```python
from build123d import *

# Parameters (mm, degrees)
SALIENTE_EXTRUIR1_DEPTH = 88.9
CROQUIS2_W              = 38.1
CROQUIS2_H              = 4.7625
CROQUIS2_W_2            = 4.7625
CROQUIS2_H_2            = 38.1
SALIENTE_EXTRUIR2_DEPTH = 76.2
CROQUIS4_R              = 6.35
CORTAR_EXTRUIR2_DEPTH   = 77.8
CROQUIS5_R              = 6.35
CORTAR_EXTRUIR3_DEPTH   = 77.8


with BuildPart() as part:
    # Croquis1 → Saliente-Extruir1 (new, symmetric)
    with BuildSketch(Plane.XY):
        Polygon((0, 31.75), (0, -31.75), (76.2, -31.75), (76.2, -26.9875), (4.7625, -26.9875), (4.7625, 26.9875), (76.2, 26.9875), (76.2, 31.75), align=None)
    extrude(amount=SALIENTE_EXTRUIR1_DEPTH, both=True)

    # Croquis2 → Saliente-Extruir2 (add, through all)
    with BuildSketch(Plane(origin=(0, 0, 0), x_dir=(0, 0, -1), z_dir=(1, 0, 0))):
        with Locations((-65.0875, 34.13125)):
            Rectangle(CROQUIS2_W, CROQUIS2_H)
        with Locations((-86.51875, 50.8)):
            Rectangle(CROQUIS2_W_2, CROQUIS2_H_2)
    saliente_extruir2 = extrude(amount=SALIENTE_EXTRUIR2_DEPTH)

    # Croquis4 → Cortar-Extruir2 (cut)
    with BuildSketch(Plane(origin=(0, 0, 84.1375), x_dir=(-1, 0, 0), z_dir=(0, 0, -1))):
        with Locations(Location((-38.1, 53.18125, 0), (0, 0, 90))):
            Circle(CROQUIS4_R)
    cortar_extruir2 = extrude(amount=-CORTAR_EXTRUIR2_DEPTH, mode=Mode.SUBTRACT)

    # Simetría3: Saliente-Extruir2, Cortar-Extruir2 across plane
    add(saliente_extruir2.mirror(Plane.ZX))
    add(cortar_extruir2.mirror(Plane.ZX), mode=Mode.SUBTRACT)

    # Croquis5 → Cortar-Extruir3 (cut)
    with BuildSketch(Plane(origin=(0, -31.75, 0), x_dir=(-1, 0, 0), z_dir=(0, -1, 0))):
        with Locations(Location((-56.2, 68.9, 0), (0, 0, 180))):
            Circle(CROQUIS5_R)
    extrude(amount=-CORTAR_EXTRUIR3_DEPTH, mode=Mode.SUBTRACT)


solid = part.part
```
For this review, take the finished solid that the model builds, in its own axes (mm). A direction names the side the tool comes from. Round coordinates to 2 decimals unless told otherwise and drop trailing zeros. Write each loop counter-clockwise with the first axis right and the second up, starting at its lowest first coordinate (ties: lowest second). Pieces come first, ordered by that corner, then holes. Notation, with made-up numbers: (62.5, -4.5) - (104.5, -4.5) arc R8 ccw to (104.5, -0.5) - close; hole circle Ø7 at (-1, 50). An arc over 180 degrees is marked (long way). Put each result on its own line as item: value.
Q1. We need section C-C (x = 21). Give the boundary of the cut face in (y, z).
Solved:
outline: (-69.85, 84.14) - (-36.51, 84.14) - (-36.51, 46.04) - (-31.75, 46.04) - (-31.75, -88.9) - (-26.99, -88.9) - (-26.99, 88.9) - (-69.85, 88.9) - close; (26.99, -88.9) - (31.75, -88.9) - (31.75, 46.04) - (36.51, 46.04) - (36.51, 84.14) - (69.85, 84.14) - (69.85, 88.9) - (26.99, 88.9) - close
Q2. Insertion check: pin 1 Ø5 at (x, y) = (22, 47.5) entering from -Z; pin 2 Ø6 at (x, z) = (36, -54) entering from +Y; pin 3 Ø23 at (x, z) = (35.5, -20.5) entering from -Y; pin 4 Ø12 at (y, z) = (8, -43) entering from -X. Each pin has a flat end and moves straight along its axis. Give the tip position at first contact, or say it passes through.
Solved:
pin 1: stops at z = 84.14
pin 2: stops at y = 31.75
pin 3: stops at y = -31.75
pin 4: stops at x = 0
Q3. Machinability: for faces 4 (the face through (39, 31.75, -20)), 5 (the face through (76.2, 31, 27)), 6 (the face through (38, -60, 84.138)), 7 (the face through (41, -26.988, 1)), which of the approach directions +Z, -Z, +X, -X, +Y, -Y give a long, thin tool a straight path to every point of the face, cutting with its end or side? Answer none if there is none.
Solved:
face 4: -Z, +X, -X, +Y
face 5: +Z, -Z, +X, +Y, -Y
face 6: -Z, +X, -X, -Y
face 7: +Z, -Z, +X
Q4. We need section A-A (x = 56.2). Give the boundary of the cut face in (y, z), and give its area (3 significant figures).
Solved:
outline: (-69.85, 84.14) - (-36.51, 84.14) - (-36.51, 46.04) - (-31.75, 46.04) - (-31.75, -62.55) - (-26.99, -62.55) - (-26.99, 88.9) - (-69.85, 88.9) - close; (-31.75, -88.9) - (-26.99, -88.9) - (-26.99, -75.25) - (-31.75, -75.25) - close; (26.99, -88.9) - (31.75, -88.9) - (31.75, -75.25) - (26.99, -75.25) - close; (26.99, -62.55) - (31.75, -62.55) - (31.75, 46.04) - (36.51, 46.04) - (36.51, 84.14) - (69.85, 84.14) - (69.85, 88.9) - (26.99, 88.9) - close
area: 2,300 mm2
Q5. Wall thickness on probe 1 along Y at (x, z) = (39, -19.5); probe 2 along Z at (x, y) = (56.2, 29.95); probe 3 along Y at (x, z) = (70, 55): over which ranges is each line inside the solid? List them lowest first.
Solved:
probe 1: y = -31.75 to -26.99, 26.99 to 31.75
probe 2: z = -88.9 to -75.25, -62.55 to 88.9
probe 3: y = -36.51 to -26.99, 26.99 to 36.51
Q6. We need section D-D (z = -48). Give the boundary of the cut face in (x, y).
Solved:
outline: (0, -31.75) - (76.2, -31.75) - (76.2, -26.99) - (4.76, -26.99) - (4.76, 26.99) - (76.2, 26.99) - (76.2, 31.75) - (0, 31.75) - close
Q7. Mouldability with a two-part tool opening along Y and no side actions: class faces 1 (the face through (0, -1, 1)), 2 (the face through (40, 26.988, 1)), 3 (the face through (38, 36.512, 65)) as released by +Y, released by -Y, zero draft, split by the parting line, or undercut.
Solved:
face 1: zero draft
face 2: undercut
face 3: released by +Y
Q8. We need section B-B (z = -68.9). Give the boundary of the cut face in (x, y).
Solved:
outline: (0, -31.75) - (49.85, -31.75) - (49.85, -26.99) - (4.76, -26.99) - (4.76, 26.99) - (49.85, 26.99) - (49.85, 31.75) - (0, 31.75) - close; (62.55, -31.75) - (76.2, -31.75) - (76.2, -26.99) - (62.55, -26.99) - close; (62.55, 26.99) - (76.2, 26.99) - (76.2, 31.75) - (62.55, 31.75) - close
